Verification items for this drawing (mm, ordinates from the low corner). A direction names the side the tool comes from. Round coordinates to 2 decimals unless told otherwise and drop trailing zeros. Order: outer loops, then holes, each group sorted by start corner. A loop starts at its lowest first (then second) coordinate and runs counter-clockwise, first axis right, second up. Notation, with made-up numbers: (11.25, 71.25) -> (46.25, 71.25) arc R21 cw to (46.25, 77.25) -> close; hole circle Ø3 at (32.5, 85.5). An arc over 180 degrees is marked (long way). Return JSON: item names as keys, results as strings. Group by question number.
Item 1: Depth check by flat-ended pin: pin 1 Ø4.5 at (x, z) = (8, 4) entering from +Y; pin 2 Ø3 at (x, z) = (8, 3) entering from +Y. Enter the tip coordinate at first touch or a pass-through.
Item 2: Sectioned sample at C-C on x = 9.75. Record the cut outline in (y, z).
Item 3: Scan lines: probe 1 along Z at (x, y) = (8, 0.8); probe 2 along Z at (x, y) = (8, 2.55); probe 3 along X at (y, z) = (3.2, 11). Record each from-to range of solid material in increasing order. Write a range as from..to.
Item 4: Sectioned sample at B-B on z = 11. Record the cut outline in (x, y), plus the area to 3 significant figures.
Item 5: Sectioned sample at A-A on x = 8. Record the cut outline in (y, z), plus the area to 3 significant figures.
Item 6: Access from +Z, -Z, +X, -X, +Y, -Y to the whole of each face (thin tool, end or side, straight path). Record for the marked faces 5 and 6.
Item 7: Draft check along X on the marked faces 1, 2, 3 and 4. Enter one of: pulls with the +X half, pulls with the -X half, needs draft (parallel to the pull), parting line crosses it, or undercut.
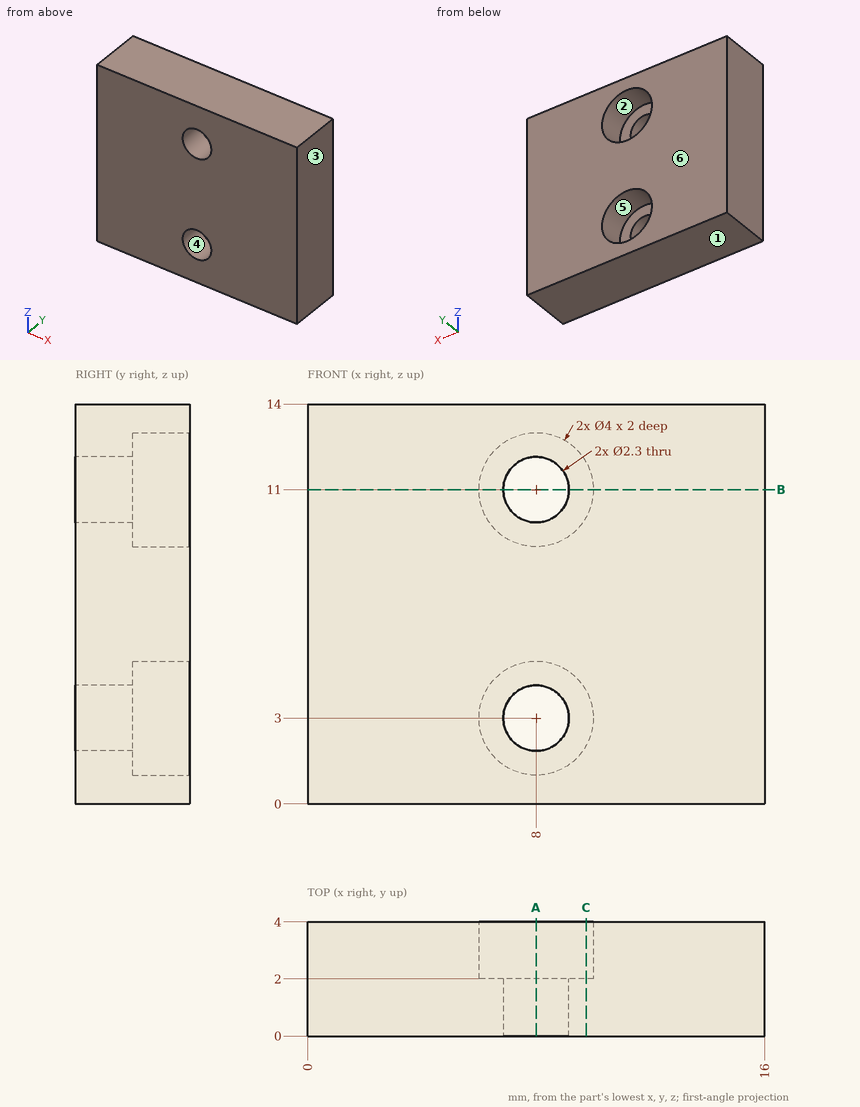
Recorded:
{
 "1": {"pin 1": "y = 4", "pin 2": "y = 2"},
 "2": {"outline": "(0, 0) -> (4, 0) -> (4, 2.03) -> (2, 2.03) -> (2, 3.97) -> (4, 3.97) -> (4, 10.03) -> (2, 10.03) -> (2, 11.97) -> (4, 11.97) -> (4, 14) -> (0, 14) -> close"},
 "3": {"probe 1": "0..1.85, 4.15..9.85, 12.15..14", "probe 2": "0..1, 5..9, 13..14", "probe 3": "0..6, 10..16"},
 "4": {"outline": "(0, 0) -> (6.85, 0) -> (6.85, 2) -> (6, 2) -> (6, 4) -> (0, 4) -> close; (9.15, 0) -> (16, 0) -> (16, 4) -> (10, 4) -> (10, 2) -> (9.15, 2) -> close", "area": "51.4 mm²"},
 "5": {"outline": "(0, 0) -> (4, 0) -> (4, 1) -> (2, 1) -> (2, 1.85) -> (0, 1.85) -> close; (0, 4.15) -> (2, 4.15) -> (2, 5) -> (4, 5) -> (4, 9) -> (2, 9) -> (2, 9.85) -> (0, 9.85) -> close; (0, 12.15) -> (2, 12.15) -> (2, 13) -> (4, 13) -> (4, 14) -> (0, 14) -> close", "area": "30.8 mm²"},
 "6": {"face 5": "+Y", "face 6": "+Z, -Z, +X, -X, +Y"},
 "7": {"face 1": "needs draft", "face 2": "undercut", "face 3": "pulls with the +X half", "face 4": "undercut"}
}
